Answer from the drawing. Dimensions are ordinates in mm from the lowest x, y and z of the part. A direction names the side the tool comes from. Coordinates: 2 decimals unless noted, no trailing zeros. Loops run counter-clockwise (first coordinate to the right, second up) from the corner with the lowest first, then second, coordinate; pieces in that order, holes last. Notation, with made-up numbers: (-4.75, -32) -> (20.25, -32) arc R7 ccw to (20.25, -23) -> close; hole circle Ø7 at (39, -30.75). An arc over 180 degrees is marked (long way). Use a Markdown table: item, result.
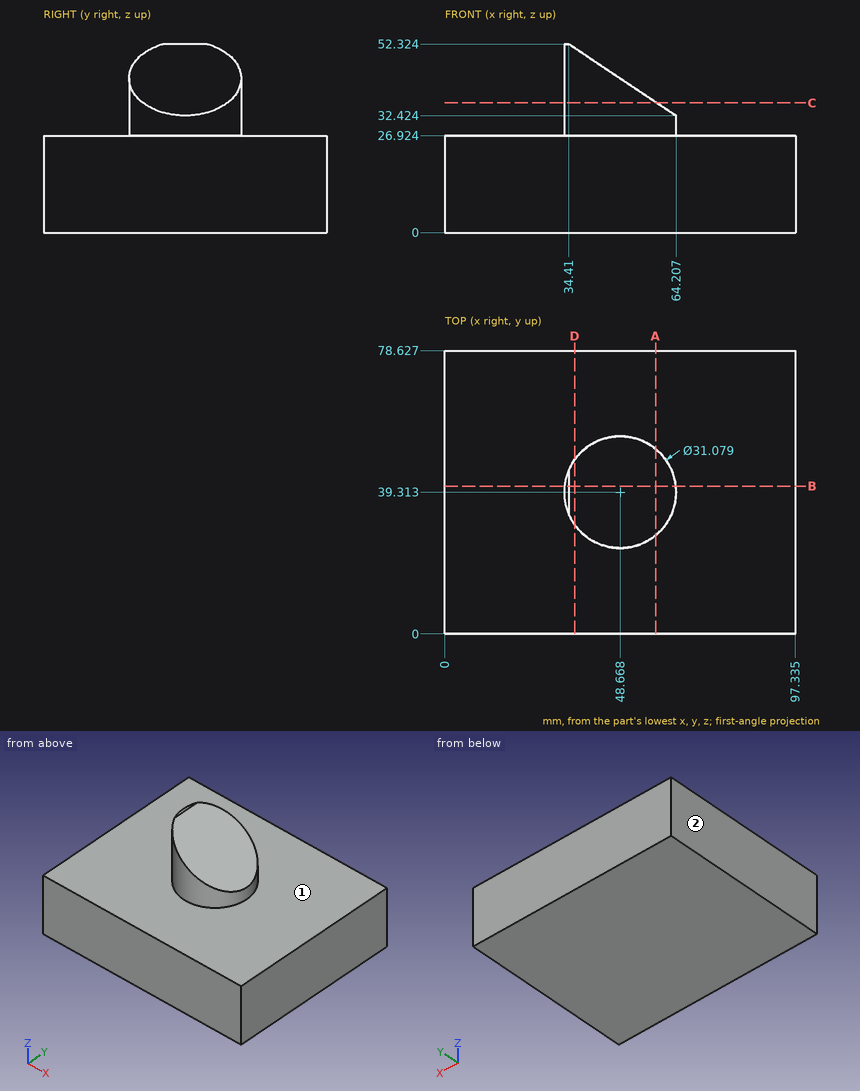
Q1. Given pin 1 Ø10 at (x, y) = (35, 68) entering from +Z; pin 2 Ø1 at (x, z) = (16, 28) entering from +Y, each flat-ended and moving along its own axis, determine where each tip first touches the part or whether it passes through.
Solved:
| item | result |
|---|---|
| pin 1 | z = 26.92 |
| pin 2 | through |
Q2. Section C-C on z = 36 is taken. Determine the outline of the cut face in (x, y).
Solved:
| item | result |
|---|---|
| outline | (58.85, 27.58) -> (58.85, 51.05) arc R15.54 ccw (long way) to start |
Q3. Section D-D on x = 36 is taken. Determine the outline of the cut face in (y, z).
Solved:
| item | result |
|---|---|
| outline | (0, 0) -> (78.63, 0) -> (78.63, 26.92) -> (48.31, 26.92) -> (48.31, 51.26) -> (30.31, 51.26) -> (30.31, 26.92) -> (0, 26.92) -> close |
Q4. Consider line 1 (Z direction, x = 27, y = 69); line 2 (Z direction, x = 55, y = 49) (1 decimal); line 3 (X direction, y = 32, z = 47) (1 decimal). Determine where each line is inside the solid, lowest interval first. Write a range as [from, to].
Solved:
| item | result |
|---|---|
| line 1 | [0, 26.92] |
| line 2 | [0, 38.6] |
| line 3 | [35, 42.4] |
Q5. Section A-A on x = 58.5 is taken. Determine the outline of the cut face in (y, z) (1 decimal).
Solved:
| item | result |
|---|---|
| outline | (0, 0) -> (78.6, 0) -> (78.6, 26.9) -> (51.3, 26.9) -> (51.3, 36.2) -> (27.3, 36.2) -> (27.3, 26.9) -> (0, 26.9) -> close |
Q6. For the marked faces 1 and 2, determine the directions among +Z, -Z, +X, -X, +Y, -Y from which every point of the face is accessible in a straight line to the end or side of a thin tool.
Solved:
| item | result |
|---|---|
| face 1 | +Z |
| face 2 | +Z, -Z, -X, +Y, -Y |
Q7. Section B-B on y = 41 is taken. Determine the outline of the cut face in (x, z) (1 decimal).
Solved:
| item | result |
|---|---|
| outline | (0, 0) -> (97.3, 0) -> (97.3, 26.9) -> (64.1, 26.9) -> (64.1, 32.5) -> (34.4, 52.3) -> (33.2, 52.3) -> (33.2, 26.9) -> (0, 26.9) -> close |
